```python
from build123d import *

# Parameters (mm, degrees)
SKETCH1_W               = 35
SKETCH1_H               = 90
BOSS_EXTRUDE1_DEPTH     = 10
SKETCH2_W               = 35
SKETCH2_H               = 10
BOSS_EXTRUDE2_DEPTH     = 40
CUT_EXTRUDE1_DEPTH      = 101.623058987
CUT_EXTRUDE1_DEPTH_BACK = 101.623058987
SKETCH3_R               = 4.090684301
SKETCH4_R               = 3.81
CUT_EXTRUDE2_DEPTH      = 105.522724802


with BuildPart() as part:
    # Sketch1 → Boss-Extrude1 (new body)
    with BuildSketch(Plane(origin=(0, 0, 0), x_dir=(1, 0, 0), z_dir=(0, 1, 0))):
        with Locations((17.5, 45)):
            Rectangle(SKETCH1_W, SKETCH1_H)
    extrude(amount=BOSS_EXTRUDE1_DEPTH)

    # Sketch2 → Boss-Extrude2 (add)
    with BuildSketch(Plane(origin=(0, 10, 0), x_dir=(1, 0, 0), z_dir=(0, 1, 0))):
        with Locations((17.5, 5)):
            Rectangle(SKETCH2_W, SKETCH2_H)
    extrude(amount=BOSS_EXTRUDE2_DEPTH)

    # Sketch3 → Cut-Extrude1 (cut, two sides: drawn at the far end of the back side and taken through both)
    with BuildSketch(Plane(origin=(0, 0, -10), x_dir=(-1, 0, 0), z_dir=(0, 0, -1)).offset(-CUT_EXTRUDE1_DEPTH_BACK)):
        with Locations((-27.5, 40)):
            Circle(SKETCH3_R)
        with Locations((-7.5, 40)):
            Circle(SKETCH3_R)
        with Locations((-7.5, 20)):
            Circle(SKETCH3_R)
        with Locations((-27.5, 20)):
            Circle(SKETCH3_R)
    extrude(amount=CUT_EXTRUDE1_DEPTH + CUT_EXTRUDE1_DEPTH_BACK, mode=Mode.SUBTRACT)

    # Sketch4 → Cut-Extrude2 (cut, through all)
    with BuildSketch(Plane(origin=(0, 10, 0), x_dir=(1, 0, 0), z_dir=(0, 1, 0))):
        with Locations(Location((17.5, 82, 0), (0, 0, 270))):
            Circle(SKETCH4_R)
    extrude(amount=-CUT_EXTRUDE2_DEPTH, mode=Mode.SUBTRACT)


solid = part.part
```
Check sheet for the modelled part. Datum: model origin and axes. Units: mm. A direction names the side the tool comes from. Give positions to 0.01 mm unless a question says otherwise; leave off trailing zeros. Write each loop counter-clockwise with the first axis right and the second up, starting at its lowest first coordinate (ties: lowest second). Pieces come first, ordered by that corner, then holes.
Item 1: Cross-section at B-B (y = 40). Enter the section's corners in (x, z).
Item 2: Cross-section at D-D (x = 7.5). Enter the section's corners in (y, z).
Item 3: Cross-section at C-C (z = -82). Enter the section's corners in (x, y), and give its area (3 significant figures).
Item 4: Access from +Z, -Z, +X, -X, +Y, -Y to the whole of each face (thin tool, end or side, straight path). Record for faces 4 (the face through (17, 10, -51)), 5 (the face through (17, 50, -5)).
Item 5: Gauge pin test, flat ends, axial feed: pin 1 (10.5 mm diameter, centred on x = 27.5, y = 20, fed in from -Z); pin 2 (9 mm diameter, centred on x = 17.5, z = -82, fed in from +Y). Record the tip position at first contact, or that the pin passes through.
Item 6: Cross-section at A-A (x = 17.5). Enter the section's corners in (y, z).
Item 7: Draft check along Y on faces 1 (the face through (17, 0, -46)), 2 (the face through (8.387, 16.007, -4.93)), 3 (the face through (35, 8, -35)). Enter one of: released by +Y, released by -Y, zero draft, split by the parting line, or undercut.
Item 8: Scan lines: L1, parallel to X at y = 40, z = -2.5; L2, parallel to Y at x = 7.5, z = -7; L3, parallel to Z at x = 31, y = 26. Record each from-to range of solid material in increasing order.
Report:
1. outline: (0, -10) - (3.41, -10) - (3.41, 0) - (0, 0) - close; (11.59, -10) - (23.41, -10) - (23.41, 0) - (11.59, 0) - close; (31.59, -10) - (35, -10) - (35, 0) - (31.59, 0) - close
2. outline: (0, -90) - (10, -90) - (10, -10) - (15.91, -10) - (15.91, 0) - (0, 0) - close; (24.09, -10) - (35.91, -10) - (35.91, 0) - (24.09, 0) - close; (44.09, -10) - (50, -10) - (50, 0) - (44.09, 0) - close
3. outline: (0, 0) - (13.69, 0) - (13.69, 10) - (0, 10) - close; (21.31, 0) - (35, 0) - (35, 10) - (21.31, 10) - close
3. area: 274 mm2
4. face 4: -Z, +X, -X, +Y
4. face 5: +Z, -Z, +X, -X, +Y
5. pin 1: stops at z = -10
5. pin 2: stops at y = 10
6. outline: (0, -90) - (10, -90) - (10, -85.81) - (0, -85.81) - close; (0, -78.19) - (10, -78.19) - (10, -10) - (50, -10) - (50, 0) - (0, 0) - close
7. face 1: released by -Y
7. face 2: undercut
7. face 3: zero draft
8. L1: x = 0 to 3.41, 11.59 to 23.41, 31.59 to 35
8. L2: y = 0 to 15.91, 24.09 to 35.91, 44.09 to 50
8. L3: z = -10 to 0
